Can you work these out from the model? Positions are in its coordinate system, mm. Face numbers are marked on the shaded views. A direction names the side the tool comes from. Round coordinates to 2 decimals unless told otherwise and drop trailing zeros. Order: outer loops, then holes, each group sorted by start corner. A loop starts at its lowest first (then second) coordinate and runs counter-clockwise, first axis right, second up.
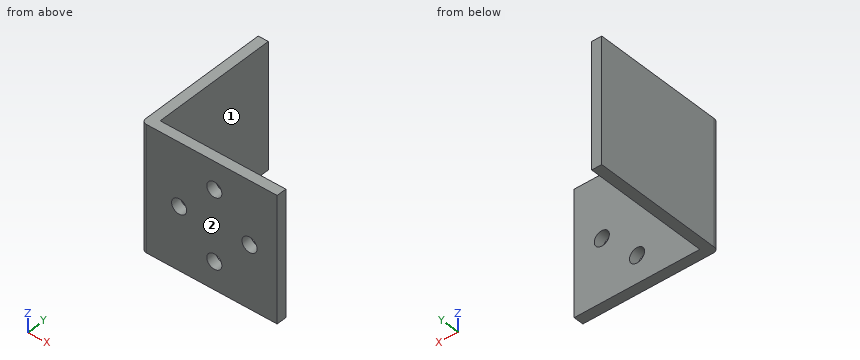
from build123d import *

# Parameters (mm, degrees)
SKETCH_1_W          = 27
SKETCH_1_H          = 25
EXTRUDE_1_DEPTH     = 2
SKETCH_2_W          = 2
SKETCH_2_H          = 25
EXTRUDE_2_DEPTH     = 25
SKETCH_3_R          = 1.5
CUT_EXTRUDE_1_DEPTH = 33.672618505
FILLET_1_R          = 1


with BuildPart() as part:
    # 草图1 → 凸台-拉伸1 (new body)
    with BuildSketch(Plane(origin=(0, 0, 0), x_dir=(1, 0, 0), z_dir=(0, 1, 0))):
        Rectangle(SKETCH_1_W, SKETCH_1_H)
    extrude(amount=EXTRUDE_1_DEPTH)

    # 草图2 → 凸台-拉伸2 (add)
    with BuildSketch(Plane(origin=(0, 2, 0), x_dir=(1, 0, 0), z_dir=(0, 1, 0))):
        with Locations((-12.5, 0)):
            Rectangle(SKETCH_2_W, SKETCH_2_H)
    extrude(amount=EXTRUDE_2_DEPTH)

    # 草图3 → 切除-拉伸1 (cut, through all)
    with BuildSketch(Plane.XZ):
        with Locations(Location((1, 7, 0), (0, 0, 270))):
            Circle(SKETCH_3_R)
        with Locations(Location((8, 0, 0), (0, 0, 270))):
            Circle(SKETCH_3_R)
        with Locations(Location((1, -7, 0), (0, 0, 270))):
            Circle(SKETCH_3_R)
        with Locations(Location((-6, 0, 0), (0, 0, 270))):
            Circle(SKETCH_3_R)
    extrude(amount=-CUT_EXTRUDE_1_DEPTH, mode=Mode.SUBTRACT)

    # 圆角1
    fillet_1_edges = [part.edges().sort_by_distance(p)[0] for p in [
        (-13.5, 0, 0),
    ]]
    fillet(fillet_1_edges, radius=FILLET_1_R)


solid = part.part
(1) I want a section at C-C, the plane z = 7. List the corners of the cut face in (x, y) for me, plus the area to 3 significant figures.
(2) I'm going to push flat-ended pins straight in: pin 1 Ø4 at (y, z) = (5, 5.5) entering from +X; pin 2 Ø4 at (x, z) = (1, 7) entering from +Y; pin 3 Ø10 at (x, y) = (-4, 4.5) entering from +Z. Where does each tip first touch, or does it pass through?
(3) Please list where these lines run through material, in increasing order: probe 1 along X at (y, z) = (0.95, 0); probe 2 along Y at (x, z) = (7, -9.5); probe 3 along X at (y, z) = (21, 1.5).
(4) On a 3-axis mill with a long thin cutter (end or side, diameter ignored), from which of +Z, -Z, +X, -X, +Y, -Y can I reach the whole of each face in a straight line? I mean the marked faces 1 and 2. Say none if no direction works.
(5) I want a section at B-B, the plane z = 0. List the corners of the cut face in (x, y) for me, plus the area to 3 significant figures.
(6) I want a section at A-A, the plane x = 1. List the corners of the cut face in (y, z) for me.
(7) I want a section at D-D, the plane x = -6. List the corners of the cut face in (y, z) for me, plus the area to 3 significant figures.
Ans:
1. outline: (-13.5, 1) arc R1 ccw to (-12.5, 0) - (-0.5, 0) - (-0.5, 2) - (-11.5, 2) - (-11.5, 27) - (-13.5, 27) - close; (2.5, 0) - (13.5, 0) - (13.5, 2) - (2.5, 2) - close
1. area: 97.8 mm2
2. pin 1: stops at x = -11.5
2. pin 2: stops at y = 2
2. pin 3: stops at z = 12.5
3. probe 1: x = -13.5 to -7.5, -4.5 to 6.5, 9.5 to 13.5
3. probe 2: y = 0 to 2
3. probe 3: x = -13.5 to -11.5
4. face 1: +Z, -Z, +X, +Y
4. face 2: +Z, -Z, +X, -X, -Y
5. outline: (-13.5, 1) arc R1 ccw to (-12.5, 0) - (-7.5, 0) - (-7.5, 2) - (-11.5, 2) - (-11.5, 27) - (-13.5, 27) - close; (-4.5, 0) - (6.5, 0) - (6.5, 2) - (-4.5, 2) - close; (9.5, 0) - (13.5, 0) - (13.5, 2) - (9.5, 2) - close
5. area: 91.8 mm2
6. outline: (0, -12.5) - (2, -12.5) - (2, -8.5) - (0, -8.5) - close; (0, -5.5) - (2, -5.5) - (2, 5.5) - (0, 5.5) - close; (0, 8.5) - (2, 8.5) - (2, 12.5) - (0, 12.5) - close
7. outline: (0, -12.5) - (2, -12.5) - (2, -1.5) - (0, -1.5) - close; (0, 1.5) - (2, 1.5) - (2, 12.5) - (0, 12.5) - close
7. area: 44.0 mm2
